Part model, mm, in its own coordinate system. Give positions to 0.01 mm unless a question says otherwise; leave off trailing zeros. Order: outer loops, then holes, each group sorted by start corner. A loop starts at its lowest first (then second) coordinate and runs counter-clockwise, first axis right, second up.
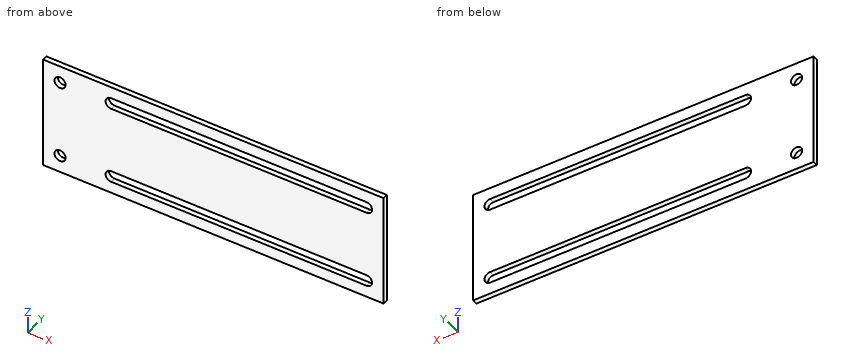
from build123d import *

# Parameters (mm, degrees)
F1_DEPTH = 3


# Not quite as in the source:
# - a feature names something its author has since deleted; it is built from what else it names


with BuildPart() as f1:
    # F0 (on Front) → F1 (new body)
    with BuildSketch(Plane.XZ):
        with BuildLine():
            Line((0, 65), (0, 55))
            Line((0, 55), (6.75, 55))
            ThreePointArc((6.75, 55), (10, 58.25), (13.25, 55))
            Line((13.25, 55), (36.75, 55))
            ThreePointArc((36.75, 55), (37.7019029611, 57.2980970389), (40, 58.25))
            Line((40, 58.25), (100, 58.25))
            Line((100, 58.25), (100, 65))
            Line((100, 65), (0, 65))
        make_face()
        with BuildLine():
            Line((0, 55), (0, 32.5))
            Line((0, 32.5), (30, 32.5))
            Line((30, 32.5), (100, 32.5))
            Line((100, 32.5), (100, 51.75))
            Line((100, 51.75), (40, 51.75))
            ThreePointArc((40, 51.75), (37.7019029611, 52.7019029611), (36.75, 55))
            Line((36.75, 55), (13.25, 55))
            ThreePointArc((13.25, 55), (10, 51.75), (6.75, 55))
            Line((6.75, 55), (0, 55))
        make_face()
        with BuildLine():
            Line((0, 32.5), (0, 10))
            Line((0, 10), (6.75, 10))
            ThreePointArc((6.75, 10), (10, 13.25), (13.25, 10))
            Line((13.25, 10), (30, 10))
            Line((30, 10), (30, 32.5))
            Line((30, 32.5), (0, 32.5))
        make_face()
        with BuildLine():
            Line((0, 10), (0, 0))
            Line((0, 0), (30, 0))
            Line((30, 0), (30, 10))
            Line((30, 10), (13.25, 10))
            ThreePointArc((13.25, 10), (10, 6.75), (6.75, 10))
            Line((6.75, 10), (0, 10))
        make_face()
        with BuildLine():
            Line((30, 32.5), (30, 10))
            Line((30, 10), (36.75, 10))
            ThreePointArc((36.75, 10), (37.7019029611, 12.2980970389), (40, 13.25))
            Line((40, 13.25), (100, 13.25))
            Line((100, 13.25), (100, 32.5))
            Line((100, 32.5), (30, 32.5))
        make_face()
        with BuildLine():
            Line((30, 10), (30, 0))
            Line((30, 0), (100, 0))
            Line((100, 0), (100, 6.75))
            Line((100, 6.75), (40, 6.75))
            ThreePointArc((40, 6.75), (37.7019029611, 7.7019029611), (36.75, 10))
            Line((36.75, 10), (30, 10))
        make_face()
        with BuildLine():
            Line((100, 32.5), (200, 32.5))
            Line((200, 32.5), (200, 65))
            Line((200, 65), (100, 65))
            Line((100, 65), (100, 58.25))
            Line((100, 58.25), (190, 58.25))
            ThreePointArc((190, 58.25), (192.2980970389, 57.2980970389), (193.25, 55))
            ThreePointArc((193.25, 55), (192.2980970389, 52.7019029611), (190, 51.75))
            Line((190, 51.75), (100, 51.75))
            Line((100, 51.75), (100, 32.5))
        make_face()
        with BuildLine():
            Line((100, 6.75), (100, 0))
            Line((100, 0), (200, 0))
            Line((200, 0), (200, 32.5))
            Line((200, 32.5), (100, 32.5))
            Line((100, 32.5), (100, 13.25))
            Line((100, 13.25), (190, 13.25))
            ThreePointArc((190, 13.25), (192.2980970389, 12.2980970389), (193.25, 10))
            ThreePointArc((193.25, 10), (192.2980970389, 7.7019029611), (190, 6.75))
            Line((190, 6.75), (100, 6.75))
        make_face()
    extrude(amount=F1_DEPTH)


solid = f1.part
Item 1: Band-saw the part on A-A on x = 132. List the corners of the cut face in (y, z).
Item 2: Drill centre lines: probe 1 along Z at (x, y) = (152.5, -2.55); probe 2 along X at (y, z) = (-1.9, 10). Where is each one in solid material? Low to high.
Item 3: Drop a flat-ended pin along its axis: P1, Ø7.5, axis at x = 10, z = 55, coming from the +Y side. Give the stop position or say it passes through.
Item 4: Band-saw the part on B-B on y = -1.7. List the corners of the cut face in (x, z).
Working result:
1. outline: (-3, 0) - (0, 0) - (0, 6.75) - (-3, 6.75) - close; (-3, 13.25) - (0, 13.25) - (0, 51.75) - (-3, 51.75) - close; (-3, 58.25) - (0, 58.25) - (0, 65) - (-3, 65) - close
2. probe 1: z = 0 to 6.75, 13.25 to 51.75, 58.25 to 65
2. probe 2: x = 0 to 6.75, 13.25 to 36.75, 193.25 to 200
3. P1: stops at y = 0
4. outline: (0, 0) - (200, 0) - (200, 65) - (0, 65) - close; hole circle Ø6.5 at (10, 10); hole circle Ø6.5 at (10, 55); hole (40, 6.75) - (190, 6.75) arc R3.25 ccw to (190, 13.25) - (40, 13.25) arc R3.25 ccw to start; hole (40, 51.75) - (190, 51.75) arc R3.25 ccw to (190, 58.25) - (40, 58.25) arc R3.25 ccw to start
